Geometry: final body of the model. Coordinates: model frame, mm. Face numbers are marked on the shaded views. Give positions to 0.01 mm unless a question says otherwise; leave off trailing zeros. Write each loop counter-clockwise with the first axis right and the second up, starting at its lowest first coordinate (ties: lowest second). Pieces come first, ordered by that corner, then holes. Notation, with made-up numbers: M -5.5,-13.75 L 51.5,-13.75 A10 cw 51.5,-1.75 Z; hole C 57.5,67 d5. An arc over 180 degrees is marked long. Use one line per item in the form item = value. Start each with the question number.
Item 1: Pull-direction query (Z, two-part tool) for the marked faces 1, 2 and 3; classes: released by +Z, released by -Z, zero draft, split by the parting line, or undercut.
Item 2: Section query A-A on x = 0. Return loops of the section in (y, z), then the cut area to 3 significant figures.
Item 3: Contact query for flat-ended pins moving along their axis: P1, Ø3, axis at x = -28, y = 69.5, coming from the -Z side; P2, Ø10, axis at x = -13, z = -54.5, coming from the +Y side; P3, Ø2, axis at x = -33, z = -92.5, coming from the -Y side. Output: stop coordinate, or through.
Item 4: Material intervals for line 1 along Z through (x, y) = (31, 186.5); line 2 along Y through (x, z) = (-1.5, -22.5); line 3 along Y through (x, z) = (11, -83), sorted ascending. Write a range as from..to.
Item 5: Section query B-B on z = -7. Return loops of the section in (x, y), then the cut area to 3 significant figures.
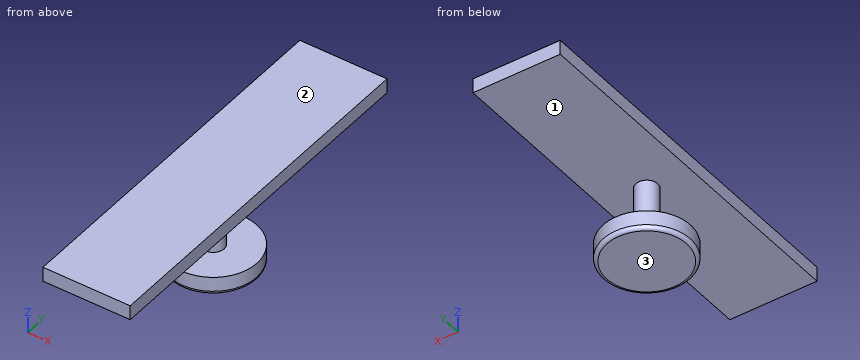
from build123d import *

# Parameters (mm, degrees)
F0_W     = 120
F0_H     = 500
F1_DEPTH = 20
F2_R     = 15
F3_DEPTH = 100
F4_R     = 60
F5_DEPTH = 25
F6_R     = 5


with BuildPart() as f1:
    # F0 (on Top) → F1 (new body)
    with BuildSketch(Plane.XY):
        Rectangle(F0_W, F0_H)
    extrude(amount=F1_DEPTH)

    # F2 (on face) → F3 (join)
    with BuildSketch(Plane.XY.offset(20)):
        with Locations((0, -3.444481)):
            Circle(F2_R)
    extrude(amount=-F3_DEPTH)

    # F4 (on face) → F5 (join)
    with BuildSketch(Plane(origin=(0, 0, -80), x_dir=(1, 0, 0), z_dir=(0, 0, -1))):
        with Locations((0, 3.444481)):
            Circle(F4_R)
    extrude(amount=F5_DEPTH)

    # F6
    f6_edges = [f1.edges().sort_by_distance(p)[0] for p in [
        (-60, -3.444481, -105),
    ]]
    fillet(f6_edges, radius=F6_R)


solid = f1.part
Answer sheet:
q1.face_1 = undercut
q1.face_2 = released by +Z
q1.face_3 = released by -Z
q2.outline = M -250,0 L -18.44,0 L -18.44,-80 L -63.44,-80 L -63.44,-100 A5 ccw -58.44,-105 L 51.56,-105 A5 ccw 56.56,-100 L 56.56,-80 L 11.56,-80 L 11.56,0 L 250,0 L 250,20 L -250,20 Z
q2.area = 15,400 mm2
q3.P1 = 0
q3.P2 = 9.24
q3.P3 = -54.2
q4.line_1 = 0..20
q4.line_2 = -18.37..11.48
q4.line_3 = -62.43..55.54
q5.outline = C 0,-3.44 d30
q5.area = 707 mm2
